The listing builds one solid part. Answer for the finished solid, in the listing's coordinates (mm). Face numbers are marked on the shaded views. A direction names the side the tool comes from. Give positions to 0.01 mm unless a question says otherwise; leave off trailing zeros. Loops run counter-clockwise (first coordinate to the right, second up) from the corner with the lowest first, then second, coordinate; pieces in that order, holes last. Notation, with made-up numbers: (80.5, 70) - (113.5, 70) arc R16 cw to (113.5, 93) - close; hole circle Ø7 at (67, 35.25). An arc over 180 degrees is marked (long way). Answer as CSV lines item,"result". Start each with the question number.
1) Flat-ended cylindrical pins translate along their axes: pin 1 (1.5 mm diameter, centred on y = 5, z = -36.5, fed in from +X); pin 2 (3 mm diameter, centred on x = 6.5, z = 0, fed in from +Y); pin 3 (1.1 mm diameter, centred on x = -6, y = 4.5, fed in from -Z). Find the tip coordinate at first contact, or state that the pin passes through.
2) A cutting plane is placed at A-A (y = 6.5). Determine the outline of the cut face in (x, z), and give its area (3 significant figures).
3) A cutting plane is placed at D-D (y = 13.5). Determine the outline of the cut face in (x, z), and give its area (3 significant figures).
4) Find the intervals of material crossed by line 1 along X through (y, z) = (15.25, 0); line 2 along X through (y, z) = (1.1, 0); line 3 along Y through (x, z) = (-17, -29), in increasing order.
5) For the marked faces 1 and 2, determine the directions among +Z, -Z, +X, -X, +Y, -Y from which every point of the face is accessible in a straight line to the end or side of a thin tool.
6) A cutting plane is placed at B-B (z = 46.25). Determine the outline of the cut face in (x, y).
```python
from build123d import *

# Parameters (mm, degrees)
BOSS_EXTRU_1_DEPTH      = 5
ENL_V_MAT_EXTRU_1_DEPTH = 15
ESQUISSE4_W             = 8
ESQUISSE4_H             = 10
ENL_V_MAT_EXTRU_2_DEPTH = 2.5
ENL_V_MAT_EXTRU_3_DEPTH = 1
ENL_V_MAT_EXTRU_4_DEPTH = 1
BOSS_EXTRU_2_DEPTH      = 5
ESQUISSE9_R             = 27.050324391
ESQUISSE9_R_2           = 23.650324391
BOSS_EXTRU_3_DEPTH      = 22
ESQUISSE10_R            = 3.42951926
ENL_V_MAT_EXTRU_5_DEPTH = 22


with BuildPart() as part:
    # Esquisse1 → Boss.-Extru.1 (new body)
    with BuildSketch(Plane(origin=(0, 0, 0), x_dir=(1, 0, 0), z_dir=(0, 1, 0))):
        with BuildLine():
            Line((-50, 55), (-10, 55))
            add(Edge.make_bspline(
                [(-10, 55), (5.148759318, 31.794007065), (43.163191576, 35.128217793), (50, 5)],
                knots=[0, 0, 0, 0, 1, 1, 1, 1], degree=3))
            Line((50, 5), (50, -55))
            Line((50, -55), (-50, -55))
            Line((-50, -55), (-50, 55))
        make_face()
    extrude(amount=BOSS_EXTRU_1_DEPTH)

    # Esquisse3 → Enlèv. mat.-Extru.1 (cut)
    with BuildSketch(Plane(origin=(0, 5, 0), x_dir=(1, 0, 0), z_dir=(0, 1, 0))):
        with BuildLine():
            Line((-38.25, 46), (-30.25, 46))
            ThreePointArc((-30.25, 46), (-28.5, 44.25), (-30.25, 42.5))
            Line((-30.25, 42.5), (-38.25, 42.5))
            ThreePointArc((-38.25, 42.5), (-40, 44.25), (-38.25, 46))
        make_face()
        with BuildLine():
            Line((-38.25, -44.5), (-30.25, -44.5))
            ThreePointArc((-30.25, -44.5), (-28.5, -46.25), (-30.25, -48))
            Line((-30.25, -48), (-38.25, -48))
            ThreePointArc((-38.25, -48), (-40, -46.25), (-38.25, -44.5))
        make_face()
        with BuildLine():
            Line((19.75, -44.5), (27.75, -44.5))
            ThreePointArc((27.75, -44.5), (29.5, -46.25), (27.75, -48))
            Line((27.75, -48), (19.75, -48))
            ThreePointArc((19.75, -48), (18, -46.25), (19.75, -44.5))
        make_face()
    extrude(amount=-ENL_V_MAT_EXTRU_1_DEPTH, mode=Mode.SUBTRACT)

    # Esquisse4 → Enlèv. mat.-Extru.2 (cut)
    with BuildSketch(Plane(origin=(0, 5, 0), x_dir=(1, 0, 0), z_dir=(0, 1, 0))):
        Rectangle(ESQUISSE4_W, ESQUISSE4_H)
    extrude(amount=-ENL_V_MAT_EXTRU_2_DEPTH, mode=Mode.SUBTRACT)

    # Esquisse6 → Enlèv. mat.-Extru.3 (cut)
    with BuildSketch(Plane(origin=(0, 5, 0), x_dir=(1, 0, 0), z_dir=(0, 1, 0))):
        with BuildLine():
            Line((-2.628313647, 16.593617601), (-3.628313647, 0.093617601))
            Line((-3.628313647, 0.093617601), (-2.628313647, -16.406382399))
            ThreePointArc((-2.628313647, -16.406382399), (-0.128313647, -18.906382399), (2.371686353, -16.406382399))
            Line((2.371686353, -16.406382399), (3.371686353, 0.093617601))
            Line((3.371686353, 0.093617601), (2.371686353, 16.593617601))
            ThreePointArc((2.371686353, 16.593617601), (-0.128313647, 19.093617601), (-2.628313647, 16.593617601))
        make_face()
    extrude(amount=-ENL_V_MAT_EXTRU_3_DEPTH, mode=Mode.SUBTRACT)

    # Esquisse7 → Enlèv. mat.-Extru.4 (cut)
    with BuildSketch(Plane(origin=(0, 5, 0), x_dir=(1, 0, 0), z_dir=(0, 1, 0))):
        with BuildLine():
            Line((-7.55, 2), (7.55, 2))
            ThreePointArc((7.55, 2), (9.55, 0), (7.55, -2))
            Line((7.55, -2), (-7.55, -2))
            ThreePointArc((-7.55, -2), (-9.55, 0), (-7.55, 2))
        make_face()
    extrude(amount=-ENL_V_MAT_EXTRU_4_DEPTH, mode=Mode.SUBTRACT)

    # Esquisse8 → Boss.-Extru.2 (add)
    with BuildSketch(Plane(origin=(0, 5, 0), x_dir=(1, 0, 0), z_dir=(0, 1, 0))):
        with BuildLine():
            Line((-2.462005123, 16.531813588), (-2.658382394, 13.291588605))
            ThreePointArc((-2.658382394, 13.291588605), (-13.493157472, 0.031813588), (-2.658382394, -13.22796143))
            Line((-2.658382394, -13.22796143), (-2.462005123, -16.468186412))
            ThreePointArc((-2.462005123, -16.468186412), (-16.650324391, 0.031813588), (-2.462005123, 16.531813588))
        make_face()
        with BuildLine():
            Line((2.537994877, 16.531813588), (2.734372149, 13.291588605))
            ThreePointArc((2.734372149, 13.291588605), (13.569147227, 0.031813588), (2.734372149, -13.22796143))
            Line((2.734372149, -13.22796143), (2.537994877, -16.468186412))
            ThreePointArc((2.537994877, -16.468186412), (16.726314146, 0.031813588), (2.537994877, 16.531813588))
        make_face()
    extrude(amount=BOSS_EXTRU_2_DEPTH)

    # Esquisse9 → Boss.-Extru.3 (add)
    with BuildSketch(Plane(origin=(0, 5, 0), x_dir=(1, 0, 0), z_dir=(0, 1, 0))):
        with Locations(Location((0, 0, 0), (0, 0, 90))):
            Circle(ESQUISSE9_R)
        with Locations(Location((0, 0, 0), (0, 0, 270))):
            Circle(ESQUISSE9_R_2, mode=Mode.SUBTRACT)
    extrude(amount=BOSS_EXTRU_3_DEPTH)

    # Esquisse10 → Enlèv. mat.-Extru.5 (cut)
    with BuildSketch(Plane(origin=(0, 2.5, 0), x_dir=(1, 0, 0), z_dir=(0, 1, 0))):
        with Locations(Location((0, 0, 0), (0, 0, 270))):
            Circle(ESQUISSE10_R)
    extrude(amount=-ENL_V_MAT_EXTRU_5_DEPTH, mode=Mode.SUBTRACT)

    # Congé1: read off the stored shape, not the designer's step
    # Congé1 outline → Congé1 (revolve, cut)
    with BuildSketch(Plane.XY):
        with BuildLine():
            ThreePointArc((23.650324391, 23.501428863), (24.640344311, 25.940691047), (27.050324391, 27))
            Line((27.050324391, 27), (23.650324391, 27))
            Line((23.650324391, 27), (23.650324391, 23.501428863))
        make_face()
    revolve(axis=Axis((0, 0, 0), (0, 1, 0)), mode=Mode.SUBTRACT)


solid = part.part
```
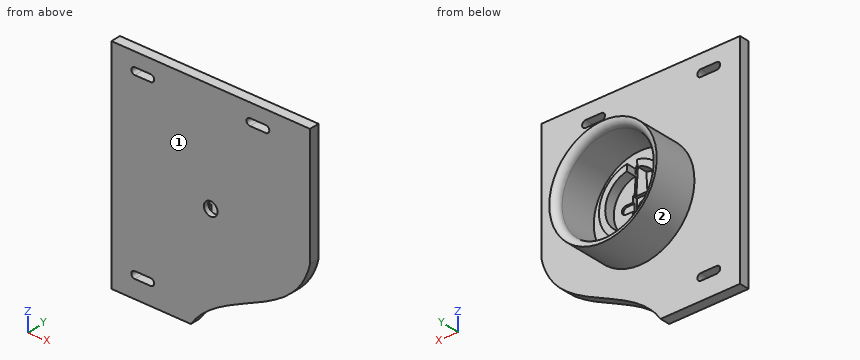
Ans:
1,pin 1,"x = 16.34"
1,pin 2,"y = 4"
1,pin 3,"z = -50.55"
2,outline,"circle Ø54.1 at (0, 0); (-2.66, -13.29) arc R13.53 cw to (-2.66, 13.23) - (-2.46, 16.47) arc R16.69 ccw to (-2.46, -16.53) - close; (2.54, -16.53) arc R16.69 ccw to (2.54, 16.47) - (2.73, 13.23) arc R13.53 cw to (2.73, -13.29) - close; hole circle Ø47.3 at (0, 0)"
2,area,"808 mm2"
3,outline,"circle Ø54.1 at (0, 0); hole circle Ø47.3 at (0, 0)"
3,area,"542 mm2"
4,line 1,"-27.05 to -23.65, 23.65 to 27.05"
4,line 2,"-50 to -3.43, 3.43 to 50"
4,line 3,"0 to 5"
5,face 1,"+Z, -Z, +X, -X, -Y"
5,face 2,"+Y"
6,outline,"(-50, 0) - (-40, 0) - (-40, 5) - (-50, 5) - close; (-28.5, 0) - (18, 0) - (18, 5) - (-28.5, 5) - close; (29.5, 0) - (50, 0) - (50, 5) - (29.5, 5) - close"
